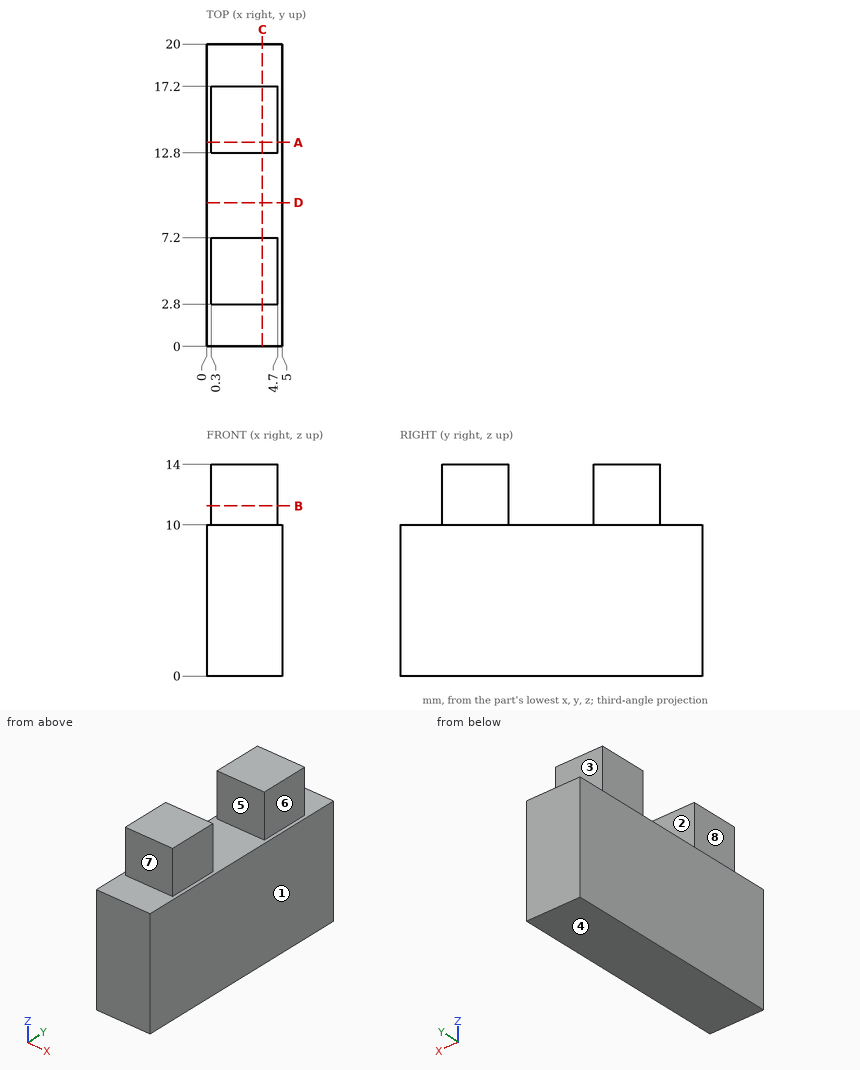
Drawing for the job (mm, zero at the part's lowest x, y, z). A direction names the side the tool comes from. Round coordinates to 2 decimals unless told otherwise and drop trailing zeros. Loops run counter-clockwise (first coordinate to the right, second up) from the corner with the lowest first, then second, coordinate; pieces in that order, holes last. Notation, with made-up numbers: (44.5, -37) -> (60.5, -37) arc R20 cw to (60.5, -26) -> close; hole circle Ø6 at (-35, 9). An arc over 180 degrees is marked (long way). Answer as CSV lines item,"result". Start each with the question number.
1) Mould opens along Y. For the marked faces 1, 2 and 3 say: +Y half, -Y half, draft (parallel to the pull), parting line (faces both ways), or undercut.
2) Tool access for the marked faces 4, 5, 6, 7 and 8: list every direction of +Z, -Z, +X, -X, +Y, -Y with a clear straight run to the whole face (end or side of a thin tool).
3) Pin check, flat tips, straight feed: P1, Ø3, axis at x = 2.5, z = 12.5, coming from the +Y side; P2, Ø3, axis at y = 15.5, z = 13, coming from the -X side; P3, Ø4.5, axis at y = 14.5, z = 11.5, coming from the +X side; P4, Ø2, axis at x = 3.5, z = 12.5, coming from the -Y side. Stop position of each tip, or through.
4) Probe line 1 along Y through (x, z) = (0.45, 13); line 2 along Z through (x, y) = (2.2, 1.75); line 3 along X through (y, z) = (14, 11.5). List the from-to ranges inside material, lowest first.
5) Slice it at A-A (y = 13.5). List the corners of the cut face in (x, z).
6) Slice it at C-C (x = 3.7). List the corners of the cut face in (y, z).
7) Slice it at B-B (z = 11.25). List the corners of the cut face in (x, y).
8) Slice it at D-D (y = 9.5). List the corners of the cut face in (x, z).
Filled in:
1,face 1,"draft"
1,face 2,"undercut"
1,face 3,"+Y half"
2,face 4,"-Z, +X, -X, +Y, -Y"
2,face 5,"+Z, +X, -X"
2,face 6,"+Z, +X, +Y, -Y"
2,face 7,"+Z, +X, -X, -Y"
2,face 8,"+Z, -X, +Y, -Y"
3,P1,"stops at y = 17.2"
3,P2,"stops at x = 0.3"
3,P3,"stops at x = 5"
3,P4,"stops at y = 2.8"
4,line 1,"y = 2.8 to 7.2, 12.8 to 17.2"
4,line 2,"z = 0 to 10"
4,line 3,"x = 0.3 to 4.7"
5,outline,"(0, 0) -> (5, 0) -> (5, 10) -> (4.7, 10) -> (4.7, 14) -> (0.3, 14) -> (0.3, 10) -> (0, 10) -> close"
6,outline,"(0, 0) -> (20, 0) -> (20, 10) -> (17.2, 10) -> (17.2, 14) -> (12.8, 14) -> (12.8, 10) -> (7.2, 10) -> (7.2, 14) -> (2.8, 14) -> (2.8, 10) -> (0, 10) -> close"
7,outline,"(0.3, 2.8) -> (4.7, 2.8) -> (4.7, 7.2) -> (0.3, 7.2) -> close; (0.3, 12.8) -> (4.7, 12.8) -> (4.7, 17.2) -> (0.3, 17.2) -> close"
8,outline,"(0, 0) -> (5, 0) -> (5, 10) -> (0, 10) -> close"
